Here's the drawing with two shaded views (mm, measured from the low corner). I have some questions. A direction names the side the tool comes from. Give positions to 0.01 mm unless a question says otherwise; leave off trailing zeros. Loops run counter-clockwise (first coordinate to the right, second up) from the corner with the lowest first, then second, coordinate; pieces in that order, holes last. Notation, with made-up numbers: M 16,84 L 75,84 A28 ccw 75,109 Z; hole C -38,57.25 d8. An arc over 180 degrees is marked long. Write item = value, one per line. Start each with the question number.
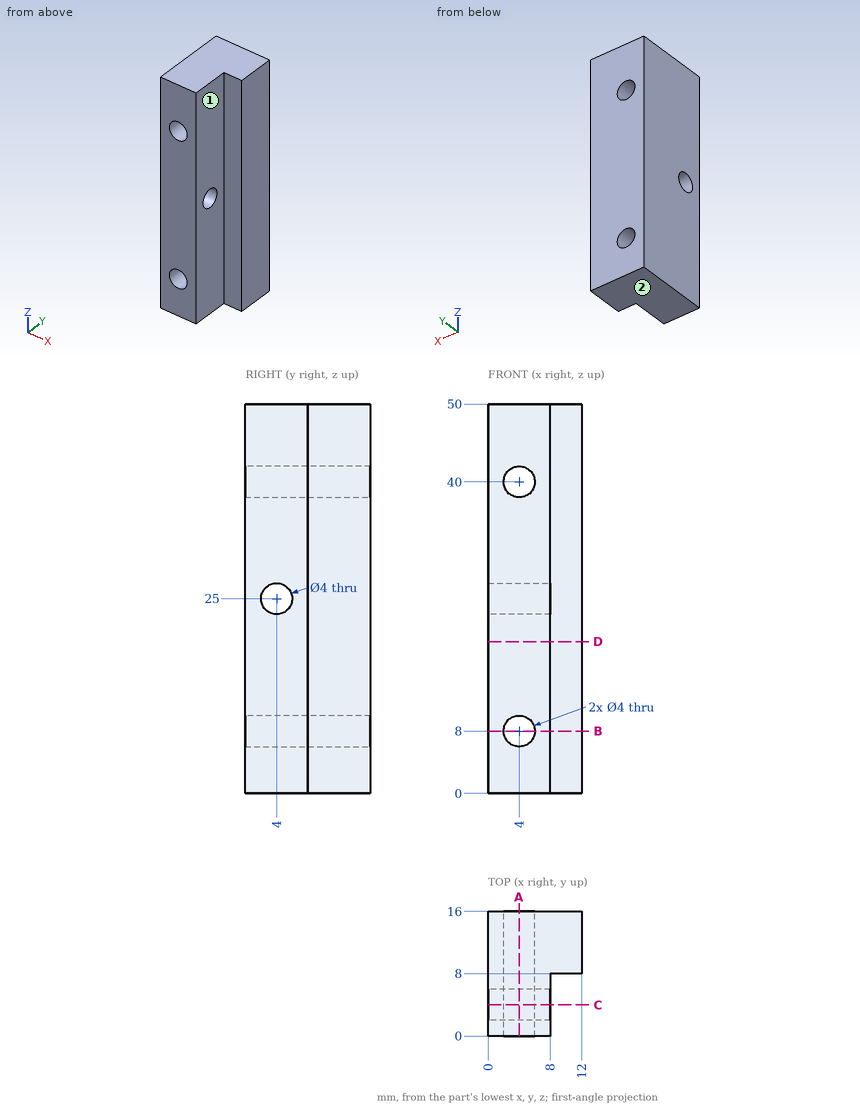
Q1. If we section it at C-C, the plane y = 4: List the corners of the cut face in (x, z) for me, then the cut area to 3 significant figures.
Q2. If I drill on line 1 along X through (y, z) = (5.75, 8); line 2 along X through (y, z) = (1, 25); line 3 along X through (y, z) = (10, 8), over which ranges is the centre line in solid material (lowest first)?
Q3. If we section it at B-B, the plane z = 8: List the corners of the cut face in (x, y) for me, then the cut area to 3 significant figures.
Q4. If we section it at D-D, the plane z = 19.5: List the corners of the cut face in (x, y) for me.
Q5. On a 3-axis mill with a long thin cutter (end or side, diameter ignored), from which of +Z, -Z, +X, -X, +Y, -Y can I reach the whole of each face in a straight line? I mean the marked faces 1 and 2. Say none if no direction works.
Q6. Will these pins go through, and if not, where does the flat tip stop? pin 1 (3.5 mm diameter, centred on y = 4, z = 25, fed in from -X); pin 2 (4 mm diameter, centred on y = 4.5, z = 37.5, fed in from +X).
Q7. If we section it at A-A, the plane x = 4: List the corners of the cut face in (y, z) for me, then the cut area to 3 significant figures.
Resolved:
q1.outline = M 0,0 L 8,0 L 8,23 L 0,23 Z; M 0,27 L 8,27 L 8,50 L 0,50 Z; hole C 4,8 d4; hole C 4,40 d4
q1.area = 343 mm²
q2.line_1 = 0 to 2, 6 to 8
q2.line_2 = 0 to 8
q2.line_3 = 0 to 2, 6 to 12
q3.outline = M 0,0 L 2,0 L 2,16 L 0,16 Z; M 6,0 L 8,0 L 8,8 L 12,8 L 12,16 L 6,16 Z
q3.area = 96.0 mm²
q4.outline = M 0,0 L 8,0 L 8,8 L 12,8 L 12,16 L 0,16 Z
q5.face_1 = +Z, -Z, +X, -Y
q5.face_2 = -Z, +X, -X, +Y, -Y
q6.pin_1 = through
q6.pin_2 = 8
q7.outline = M 0,0 L 16,0 L 16,6 L 0,6 Z; M 0,10 L 16,10 L 16,38 L 0,38 Z; M 0,42 L 16,42 L 16,50 L 0,50 Z; hole C 4,25 d4
q7.area = 659 mm²
